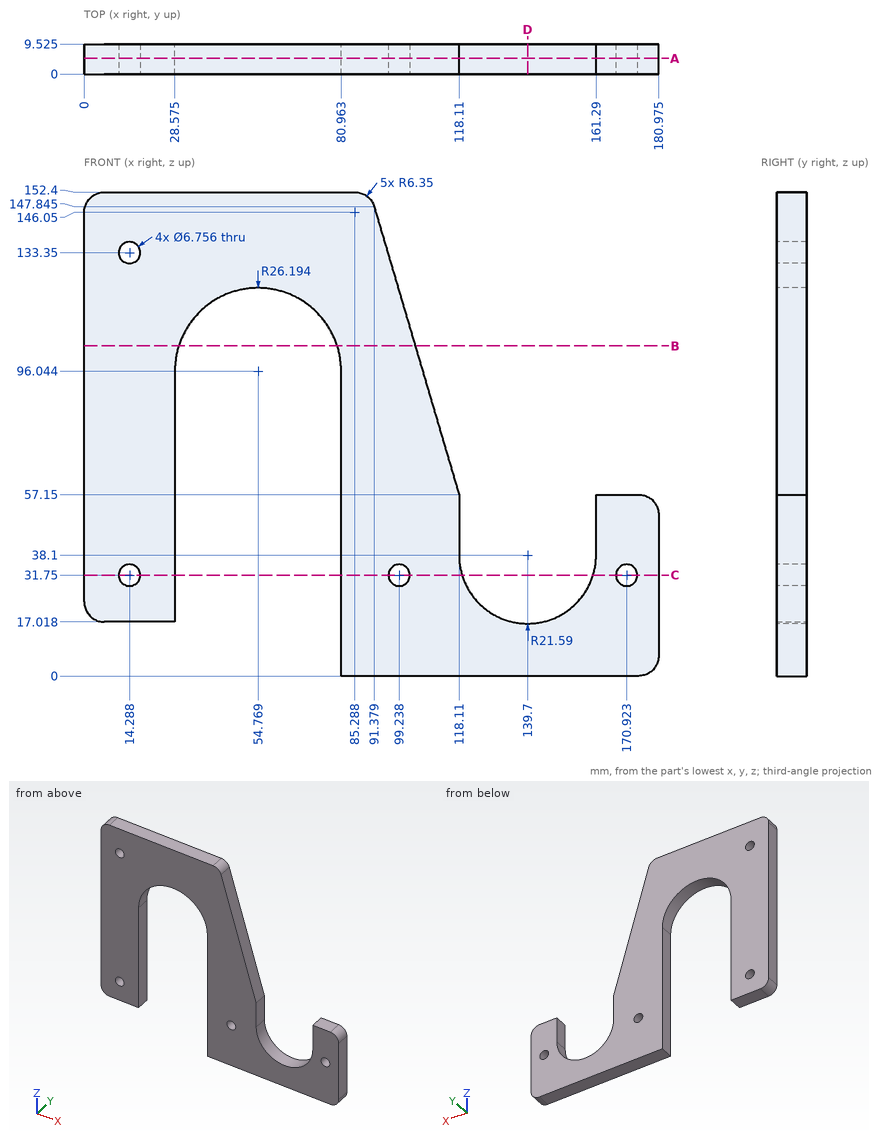
Answer from the drawing. Dimensions are ordinates in mm from the lowest x, y and z of the part. Round coordinates to 2 decimals unless told otherwise and drop trailing zeros. Write each loop counter-clockwise with the first axis right and the second up, starting at its lowest first coordinate (ties: lowest second). Pieces come first, ordered by that corner, then holes. Notation, with made-up numbers: (44.25, 75) - (51.25, 75) arc R22 ccw to (51.25, 102) - close; hole circle Ø2 at (-32.5, 81). An arc over 180 degrees is marked (long way). One line per item, written item: value.
Q1. Find section C-C (z = 31.75). Determine the outline of the cut face in (x, y) (1 decimal).
The answers:
outline: (0, 0) - (10.9, 0) - (10.9, 9.5) - (0, 9.5) - close; (17.7, 0) - (28.6, 0) - (28.6, 9.5) - (17.7, 9.5) - close; (81, 0) - (95.9, 0) - (95.9, 9.5) - (81, 9.5) - close; (102.6, 0) - (119.1, 0) - (119.1, 9.5) - (102.6, 9.5) - close; (160.3, 0) - (167.5, 0) - (167.5, 9.5) - (160.3, 9.5) - close; (174.3, 0) - (181, 0) - (181, 9.5) - (174.3, 9.5) - close
Q2. Straight lines are drawn through the part: line 1 (X direction, y = 1.25, z = 41) (1 decimal); line 2 (X direction, y = 5, z = 54.5) (1 decimal); line 3 (X direction, y = 6, z = 31.75) (1 decimal). For each, find the intervals that lie inside material, in ascending order. Write a range as from..to.
The answers:
line 1: x = 0..28.6, 81..118.1, 161.3..181
line 2: x = 0..28.6, 81..118.1, 161.3..179.8
line 3: x = 0..10.9, 17.7..28.6, 81..95.9, 102.6..119.1, 160.3..167.5, 174.3..181
Q3. Find section A-A (y = 5). Count the separate pieces of the cut face and the enclosed holes in it, and give its area (3 significant figures).
The answers:
separate pieces: 1
enclosed holes: 4
area: 11,900 mm2
Q4. Each of these flat-tipped pins is pushed along its axis until it touches: P1, Ø1, axis at y = 5, z = 124, coming from the +X side (1 decimal); P2, Ø4, axis at y = 8, z = 131.5, coming from the +X side (1 decimal); P3, Ø5, axis at x = 13.5, y = 4.5, coming from the -Z side. Where does it stop, or does it pass through?
The answers:
P1: stops at x = 98.6
P2: stops at x = 96.8
P3: stops at z = 17.02
Q5. Find section D-D (x = 139.7). Determine the outline of the cut face in (y, z) (1 decimal), and give its area (3 significant figures).
The answers:
outline: (0, 0) - (9.5, 0) - (9.5, 16.5) - (0, 16.5) - close
area: 157 mm2
Q6. Find section B-B (z = 104). Determine the outline of the cut face in (x, y) (1 decimal), and give its area (3 significant figures).
The answers:
outline: (0, 0) - (29.8, 0) - (29.8, 9.5) - (0, 9.5) - close; (79.7, 0) - (104.3, 0) - (104.3, 9.5) - (79.7, 9.5) - close
area: 518 mm2
